Answer from the drawing. Dimensions are ordinates in mm from the lowest x, y and z of the part. Round coordinates to 2 decimals unless told otherwise and drop trailing zeros. Loops run counter-clockwise (first coordinate to the right, second up) from the corner with the lowest first, then second, coordinate; pieces in that order, holes last. Notation, with made-up numbers: (28, 13.5) - (56, 13.5) arc R20 cw to (56, 39.5) - close; hole circle Ø11 at (-34.5, 43). An arc over 180 degrees is marked (long way). Return JSON: item names as keys, results as strings.
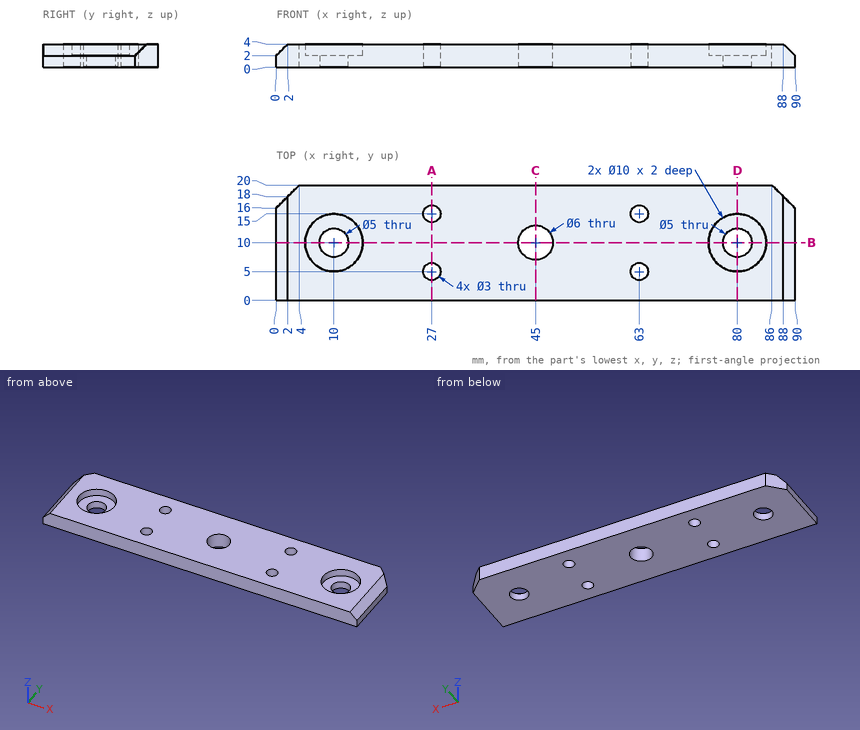
1) Find the intervals of material crossed by L1, parallel to X at y = 10, z = 0.6; L2, parallel to Y at x = 63, z = 1.5; L3, parallel to X at y = 10.5, z = 3.75, in increasing order.
Verdict:
{"L1": "x = 0 to 7.5, 12.5 to 42, 48 to 77.5, 82.5 to 90", "L2": "y = 0 to 3.5, 6.5 to 13.5, 16.5 to 20", "L3": "x = 1.75 to 5.03, 14.97 to 42.04, 47.96 to 75.03, 84.97 to 88.25"}
2) Section A-A (x = 27) is taken. Give the vertices of the cut face in (y, z), and give its area (3 significant figures).
Verdict:
{"outline": "(0, 0) - (3.5, 0) - (3.5, 4) - (0, 4) - close; (6.5, 0) - (13.5, 0) - (13.5, 4) - (6.5, 4) - close; (16.5, 0) - (20, 0) - (20, 4) - (16.5, 4) - close", "area": "56.0 mm2"}
3) Section D-D (x = 80) is taken. Give the vertices of the cut face in (y, z).
Verdict:
{"outline": "(0, 0) - (7.5, 0) - (7.5, 2) - (5, 2) - (5, 4) - (0, 4) - close; (12.5, 0) - (20, 0) - (20, 4) - (15, 4) - (15, 2) - (12.5, 2) - close"}
4) Section C-C (x = 45) is taken. Give the vertices of the cut face in (y, z).
Verdict:
{"outline": "(0, 0) - (7, 0) - (7, 4) - (0, 4) - close; (13, 0) - (20, 0) - (20, 4) - (13, 4) - close"}
5) Flat-ended cylindrical pins translate along their axes: pin 1 (2.5 mm diameter, centred on x = 27, y = 15, fed in from +Z); pin 2 (6 mm diameter, centred on x = 10, y = 10, fed in from +Z). Find the tip coordinate at first contact, or state that the pin passes through.
Verdict:
{"pin 1": "passes through", "pin 2": "stops at z = 2"}
6) Section B-B (y = 10) is taken. Give the vertices of the cut face in (x, z), and give its area (3 significant figures).
Verdict:
{"outline": "(0, 0) - (7.5, 0) - (7.5, 2) - (5, 2) - (5, 4) - (2, 4) - (0, 2) - close; (12.5, 0) - (42, 0) - (42, 4) - (15, 4) - (15, 2) - (12.5, 2) - close; (48, 0) - (77.5, 0) - (77.5, 2) - (75, 2) - (75, 4) - (48, 4) - close; (82.5, 0) - (90, 0) - (90, 2) - (88, 4) - (85, 4) - (85, 2) - (82.5, 2) - close", "area": "272 mm2"}
